Autodesk Inventor part; units mm, degrees
ref_plane "Work Plane1" through (-11.8839, 0, 1.1821) normal (-0.0989806, 0, -0.9950894) x (0, -1, 0)
ref_plane "YZ Plane" through (0, 0, 0) normal (1, 0, 0) x (0, 1, 0)
ref_plane "XZ Plane" through (0, 0, 0) normal (0, 1, 0) x (-1, 0, 0)
sketch "Sketch1" plane through (0, 0, 0) normal (0, 1, 0) x (-1, 0, 0)
  arc A0 (11.8839, 1.1821) -> (-11.8839, 1.1821) centre (0, 0) ccw
  arc A1 (-23.7682, -118.2958) -> (23.7682, -118.2958) centre (0, -120.66) ccw
  line L0 (11.8839, 1.1821) -> (23.7682, -118.2958)
  line L1 (-11.8839, 1.1821) -> (-23.7682, -118.2958)
  dimension "d0" = 23.885
  dimension "d1" = 47.771
  dimension "d2" = 120.66
ref_plane "Work Plane1" through (-11.8839, 0, 1.1821) normal (-0.0989806, 0, -0.9950894) x (0, -1, 0)
sketch "Sketch2" plane through (-11.8839, 0, 1.1821) normal (-0.0989806, 0, -0.9950894) x (0, -1, 0)
  line L0 (-7.5, 1.2) -> (7.5, 1.2)
  line L1 (7.5, 1.2) -> (7.5, 0)
  line L2 (7.5, 0) -> (-7.5, 0)
  line L3 (-7.5, 0) -> (-7.5, 1.2)
  line L4 (-7.5, 1.2) -> (7.5, 0) construction
  line L5 (7.5, 1.2) -> (-7.5, 0) construction
  point P0 (0, -11.9425)
  point P1 (0, 0.6)
  point P2 (0, 0)
  point P3 (0, 0)
  dimension "d3" = 1.2
  dimension "d4" = 15
sweep "Sweep1" add profiles "Sketch2" path "Sketch1"
properties part number "2309HCMUTE-CDT23-BELT_S5M-355X71X15" material "Rubber"
CAD build for the part. Positions are in the model's coordinates, mm. A direction names the side the tool comes from. Coordinates: 2 decimals unless noted, no trailing zeros. Order: outer loops, then holes, each group sorted by start corner. A loop starts at its lowest first (then second) coordinate and runs counter-clockwise, first axis right, second up.
Item 1: Drill centre lines: L1, parallel to Z at x = 0.5, y = 0.75; L2, parallel to X at y = 3.25, z = -120.66; L3, parallel to X at y = 3.25, z = -4. Where is each one in solid material? Low to high.
Check sheet entries:
L1: z = -145.74 to -144.54, 11.93 to 13.13
L2: x = -25.09 to -23.89, 23.89 to 25.09
L3: x = -13.61 to -12.4, 12.4 to 13.61
Item 2: Band-saw the part on B-B on z = -120.66. List the corners of the cut face in (x, y), plus the area to 3 significant figures.
Check sheet entries:
outline: (-25.09, -7.5) - (-23.89, -7.5) - (-23.89, 7.5) - (-25.09, 7.5) - close; (23.89, -7.5) - (25.09, -7.5) - (25.09, 7.5) - (23.89, 7.5) - close
area: 36.0 mm2
Item 3: Two-plate mould, pull along Z, no slides. Class faces 3 (the face through (-17.743, 0.105, -57.721)), 4 (the face through (-0.27, 0.11, 13.14)), 5 (the face through (-20, -7.5, -73)): +Z half, -Z half, draft (parallel to the pull), parting line (faces both ways), or undercut.
Check sheet entries:
face 3: undercut
face 4: +Z half
face 5: draft
Item 4: 3-axis set-ups, long thin cutter, end or side, ignore diameter. For faces 1 (the face through (19.103, -0.105, -59.274)), 2 (the face through (17.91, 0.1, -59.39)): which of +Z, -Z, +X, -X, +Y, -Y reach the whole face in a straight line?
Check sheet entries:
face 1: +Z, +X, +Y, -Y
face 2: +Y, -Y
Item 5: Band-saw the part on C-C on y = -5. List the corners of the cut face in (x, z).
Check sheet entries:
outline: (-24.96, -118.18) arc R25.09 ccw (long way) to (24.96, -118.18) - (13.08, 1.3) arc R13.14 ccw to (-13.08, 1.3) - close; hole (-23.77, -118.3) arc R23.89 ccw (long way) to (23.77, -118.3) - (11.88, 1.18) arc R11.94 ccw to (-11.88, 1.18) - close
Item 6: Pin check, flat tips, straight feed: pin 1 Ø1 at (y, z) = (-1, -80) entering from +X; pin 2 Ø8 at (y, z) = (2.5, -79.5) entering from -X; pin 3 Ø5 at (y, z) = (-2, -40) entering from -X. Stop position of each tip, or through.
Check sheet entries:
pin 1: stops at x = 21.21
pin 2: stops at x = -21.51
pin 3: stops at x = -17.43
Item 7: Band-saw the part on A-A on x = 0. List the corners of the cut face in (y, z), plus the area to 3 significant figures.
Check sheet entries:
outline: (-7.5, -145.75) - (7.5, -145.75) - (7.5, -144.55) - (-7.5, -144.55) - close; (-7.5, 11.94) - (7.5, 11.94) - (7.5, 13.14) - (-7.5, 13.14) - close
area: 36.0 mm2
